from build123d import *

# Parameters (mm, degrees)
EXTRUDE_1_DEPTH = 10


with BuildPart() as part:
    # Эскиз1 → Бобышка-Вытянуть1 (new body)
    with BuildSketch(Plane.XY):
        Polygon((-66.282586336, 4.09041909), (-74.040470763, 8.357255525), (-70.161528549, 11.848303517), (-66.282586336, 15.339351509), (-66.282586336, 19.218293722), (-75.209365057, 24.128022019), (-60.314226958, 24.128022019), (-70.745975697, 35.71885395), (-67.761796008, 38.40461567), (-55.730109265, 38.40461567), (-61.745952636, 48.606953693), (-52.460988202, 52.175342696), (-43.416291781, 45.665500099), (-46.838743542, 54.570735165), (-41.684369065, 57.610029636), (-37.461610157, 54.570735165), (-34.477282264, 59.996785881), (-23.420274879, 59.996785881), (-20.22078559, 54.570735165), (-17.236457696, 59.996785881), (-1.763387891, 59.996785881), (12.653887704, 54.570735165), (16.559241123, 59.996785881), (26.230185451, 59.996785881), (34.710427131, 53.893204737), (51.197564442, 56.580039943), (56.124240189, 53.034107371), (56.124240189, 45.665500099), (66.212425028, 38.40461567), (63.264526212, 26.381057915), (69.711013986, 19.218293722), (67.048138131, 8.357255525), (70.712863391, 2.142205771), (61.168332609, 2.142205771), (70.712863391, -4.727388317), (64.73847562, -8.250206419), (64.73847562, -13.02813029), (61.735677356, -21.006708523), (58.995962435, -21.006708523), (63.237076488, -28.199262665), (61.116519462, -33.833683844), (53.138381044, -44.918412685), (42.953995786, -50.923670147), (34.710427131, -50.923670147), (21.394713287, -50.923670147), (12.653887704, -44.632535977), (-1.763387891, -41.097752801), (-17.236457696, -41.097752801), (-39.572989611, -41.097752801), (-55.730109265, -39.376048265), (-65.530101327, -39.376048265), (-74.040470763, -38.469182314), (-68.6764474, -31.016473255), (-72.590645655, -28.199262665), (-72.590645655, -19.765075522), (-72.590645655, -11.813243984), (-72.590645655, -8.250206419), (-72.590645655, 2.142205771), align=None)
    extrude(amount=EXTRUDE_1_DEPTH)


solid = part.part
CAD build for the part. Positions are in the model's coordinates, mm. A direction names the side the tool comes from. Give positions to 0.01 mm unless a question says otherwise; leave off trailing zeros. Write each loop counter-clockwise with the first axis right and the second up, starting at its lowest first coordinate (ties: lowest second). Pieces come first, ordered by that corner, then holes. Notation, with made-up numbers: (17, 34.25) -> (56, 34.25) arc R15 cw to (56, 61.25) -> close; hole circle Ø2 at (15.25, 2.5). An arc over 180 degrees is marked (long way). Return JSON: item names as keys, results as strings.
Item 1: Drill centre lines: probe 1 along Y at (x, z) = (-57.5, 3); probe 2 along Y at (x, z) = (-35, 8.25); probe 3 along X at (y, z) = (1, 9). Where is each one in solid material? Low to high.
Answer below:
{"probe 1": "y = -39.38 to 38.4, 41.41 to 50.24", "probe 2": "y = -41.1 to 59.05", "probe 3": "x = -72.59 to 62.76"}
Item 2: Band-saw the part on A-A (x = 46.5). List the corners of the cut face in (y, z).
Answer below:
{"outline": "(-48.83, 0) -> (55.81, 0) -> (55.81, 10) -> (-48.83, 10) -> close"}
Item 3: Tool access for faces 5 (the flat face through (-65.457, 29.842, 4.93)), 6 (the flat face through (-21, -41.098, 5)), 7 (the flat face through (30.41, 56.99, 4.93)): list every direction of +Z, -Z, +X, -X, +Y, -Y with a clear straight run to the whole face (end or side of a thin tool).
Answer below:
{"face 5": "+Z, -Z, -X", "face 6": "+Z, -Z, -X, -Y", "face 7": "+Z, -Z, +Y"}
Item 4: Two-plate mould, pull along Y, no slides. Class faces 1 (the flat face through (-70.606, -29.628, 4.93)), 2 (the flat face through (-35.99, 57.25, 4.93)), 3 (the flat face through (17.085, -47.822, 4.93)), 4 (the flat face through (61.087, -24.553, 4.93)): +Y half, -Y half, draft (parallel to the pull), parting line (faces both ways), or undercut.
Answer below:
{"face 1": "undercut", "face 2": "+Y half", "face 3": "-Y half", "face 4": "undercut"}
Item 5: Drop flat-ended pins along their axis: pin 1 (1 mm diameter, centred on y = -36.5, z = 7.5, fed in from +X); pin 2 (5 mm diameter, centred on x = -65.5, z = 5.5, fed in from +Y); pin 3 (5 mm diameter, centred on x = -27.5, z = 7, fed in from -Y). Give the stop position or say it passes through.
Answer below:
{"pin 1": "stops at x = 59.56", "pin 2": "stops at y = 38.4", "pin 3": "stops at y = -41.1"}
Item 6: Band-saw the part on B-B (y = 17.5). List the corners of the cut face in (x, z).
Answer below:
{"outline": "(-66.28, 0) -> (69.29, 0) -> (69.29, 10) -> (-66.28, 10) -> close"}
